Design review of the part built by this model. Coordinates are the model's own, in mm. A direction names the side the tool comes from. Give positions to 0.01 mm unless a question says otherwise; leave off trailing zeros. Write each loop counter-clockwise with the first axis right and the second up, starting at its lowest first coordinate (ties: lowest second). Pieces come first, ordered by that corner, then holes. Notation, with made-up numbers: (22, -34) -> (67, -34) arc R19 ccw to (67, -30) -> close; hole circle Ø2 at (69, -8). An arc over 180 degrees is marked (long way). Use CSV: the item, a comma, the result in double quotes.
```python
from build123d import *

# Parameters (mm, degrees)
SKETCH1_R           = 2.7
BOSS_EXTRUDE1_DEPTH = 3
BOSS_EXTRUDE2_DEPTH = 3
CUT_EXTRUDE1_DEPTH  = 3
FILLET1_R           = 4
FILLET2_R           = 2
FILLET3_R           = 1


with BuildPart() as part:
    # Sketch1 → Boss-Extrude1 (new body)
    with BuildSketch(Plane.XY):
        Polygon((0, 0), (0, 15), (50, 15), (50, -43), (31, -43), (31, 0), align=None)
        with Locations((7, 9)):
            Circle(SKETCH1_R, mode=Mode.SUBTRACT)
    extrude(amount=-BOSS_EXTRUDE1_DEPTH)

    # Sketch2 → Boss-Extrude2 (add)
    with BuildSketch(Plane(origin=(0, 0, -3), x_dir=(-1, 0, 0), z_dir=(0, 0, -1))):
        Polygon((-50, 15), (-50, 9), (-37, 9), (-37, -37), (-50, -37), (-50, -43), (-31, -43), (-31, 15), align=None)
    extrude(amount=BOSS_EXTRUDE2_DEPTH)

    # Sketch3 → Cut-Extrude1 (cut)
    with BuildSketch(Plane.XY):
        with BuildLine():
            Line((41, -17.5), (50, -17.5))
            Line((50, -17.5), (50, -24.5))
            Line((50, -24.5), (41, -24.5))
            ThreePointArc((41, -24.5), (37.5, -21), (41, -17.5))
        make_face()
    extrude(amount=-CUT_EXTRUDE1_DEPTH, mode=Mode.SUBTRACT)

    # Fillet1
    fillet1_edges = [part.edges().sort_by_distance(p)[0] for p in [
        (0, 0, -1.5),
        (0, 15, -1.5),
    ]]
    fillet(fillet1_edges, radius=FILLET1_R)

    # Fillet2
    fillet2_edges = [part.edges().sort_by_distance(p)[0] for p in [
        (50, -17.5, -1.5),
        (50, -24.5, -1.5),
    ]]
    fillet(fillet2_edges, radius=FILLET2_R)

    # Fillet3
    fillet3_edges = [part.edges().sort_by_distance(p)[0] for p in [
        (50, 15, -3),
        (50, -43, -3),
        (31, -43, -3),
        (31, 15, -4.5),
    ]]
    fillet(fillet3_edges, radius=FILLET3_R)


solid = part.part
```
(1) For line 1 along Y through (x, z) = (41, -0.95); line 2 along Y through (x, z) = (7, -1.65); line 3 along Y through (x, z) = (11, -2.9), list the stretches that pass through material, from the lowest coordinate up. Write a range as [from, to].
Established:
line 1,"y = [-43, -24.5], [-17.5, 15]"
line 2,"y = [0, 6.3], [11.7, 15]"
line 3,"y = [0, 15]"
(2) Take a section at A-A (x = 7). Write out the cut boundary in (y, z), then the cut area to 3 significant figures.
Established:
outline,"(0, -3) -> (6.3, -3) -> (6.3, 0) -> (0, 0) -> close; (11.7, -3) -> (15, -3) -> (15, 0) -> (11.7, 0) -> close"
area,"28.8 mm2"
(3) Take a section at D-D (y = 7). Write out the cut boundary in (x, z), then the cut area to 3 significant figures.
Established:
outline,"(0, -3) -> (5.19, -3) -> (5.19, 0) -> (0, 0) -> close; (8.81, -3) -> (31, -3) -> (31, -6) -> (37, -6) -> (37, -3) -> (50, -3) -> (50, 0) -> (8.81, 0) -> close"
area,"157 mm2"
(4) Take a section at C-C (y = -1). Write out the cut boundary in (x, z), then the cut area to 3 significant figures.
Established:
outline,"(31, -6) -> (37, -6) -> (37, -3) -> (50, -3) -> (50, 0) -> (31, 0) -> close"
area,"75.0 mm2"
(5) Take a section at B-B (z = -1.6). Write out the cut boundary in (x, y).
Established:
outline,"(0, 4) arc R4 ccw to (4, 0) -> (31, 0) -> (31, -42) arc R1 ccw to (32, -43) -> (49, -43) arc R1 ccw to (50, -42) -> (50, -26.5) arc R2 ccw to (48, -24.5) -> (41, -24.5) arc R3.5 cw to (41, -17.5) -> (48, -17.5) arc R2 ccw to (50, -15.5) -> (50, 14) arc R1 ccw to (49, 15) -> (4, 15) arc R4 ccw to (0, 11) -> close; hole circle Ø5.4 at (7, 9)"
(6) Mouldability with a two-part tool opening along Y and no side actions: class faces 4 (the face through (50, 3, -2)), 5 (the face through (1.203, 13.859, -1.521)), 6 (the face through (18, 0, -1)), 7 (the face through (44, -14, -3)) as +Y half, -Y half, draft (parallel to the pull), parting line (faces both ways), or undercut.
Established:
face 4,"draft"
face 5,"+Y half"
face 6,"-Y half"
face 7,"undercut"
(7) Clearance check with flat-ended pins moving along their axes: pin 1 (12 mm diameter, centred on x = 10, y = 10, fed in from -Z); pin 2 (1.5 mm diameter, centred on y = -23, z = -4, fed in from +X); pin 3 (2.5 mm diameter, centred on x = 19.5, z = -1.5, fed in from -Y). State where each tip first meets the part, or that it passes through.
Established:
pin 1,"stops at z = -3"
pin 2,"stops at x = 37"
pin 3,"stops at y = 0"
(8) Tool access review of faces 1 (the face through (49.43, -25.1, -1.52)), 2 (the face through (31, 15, -2)), 3 (the face through (43, -37, -4)): name each direction out of +Z, -Z, +X, -X, +Y, -Y from which nothing blocks a thin tool from reaching the whole face with its end or side.
Established:
face 1,"+Z, -Z, +X"
face 2,"+Z, -Z, +X, -X, +Y"
face 3,"-Z, +X"
